Can you work these out from the model? Positions are in its coordinate system, mm. A direction names the side the tool comes from. Give positions to 0.01 mm unless a question says otherwise; leave off trailing zeros. Loops run counter-clockwise (first coordinate to the right, second up) from the corner with the lowest first, then second, coordinate; pieces in that order, holes last. Notation, with made-up numbers: (5.25, 29.5) - (13.25, 29.5) arc R25 cw to (13.25, 51.5) - close; hole circle Ø10 at (-22, -10). An arc over 180 degrees is marked (long way). Write item = value, one per line.
from build123d import *

# Parameters (mm, degrees)
SKETCH_31_W              = 56.5
SKETCH_31_H              = 38
EXTRUDE_11_DEPTH         = 4
SKETCH_32_W              = 4
SKETCH_32_H              = 38
EXTRUDE_12_DEPTH         = 29.5
SKETCH_33_W              = 16
SKETCH_33_H              = 38
EXTRUDE_13_DEPTH         = 4
SKETCH_34_W              = 15
SKETCH_34_H              = 4
EXTRUDE_14_DEPTH         = 29.5
HOLE_WIZARD_M2_5_1_D     = 2.9
HOLE_WIZARD_M2_5_1_DEPTH = 10
HOLE_WIZARD_M2_5_1_TIP   = 0.871247898
HOLE_WIZARD_M2_5_2_D     = 2.9
HOLE_WIZARD_M2_5_2_DEPTH = 10
HOLE_WIZARD_M2_5_2_TIP   = 0.871247898
HOLE_WIZARD_M2_5_3_D     = 2.9
HOLE_WIZARD_M2_5_3_DEPTH = 10
HOLE_WIZARD_M2_5_3_TIP   = 0.871247898
HOLE_WIZARD_M4_1_D       = 4.5
HOLE_WIZARD_M4_1_DEPTH   = 10
HOLE_WIZARD_M4_1_TIP     = 1.351936393
SKETCH_46_W              = 43
SKETCH_46_H              = 33.5
CUT_EXTRUDE_4_DEPTH      = 4


with BuildPart() as part:
    # 스케치31 → 보스-돌출11 (new body)
    with BuildSketch(Plane(origin=(0, 0, 0), x_dir=(1, 0, 0), z_dir=(0, 1, 0))):
        Rectangle(SKETCH_31_W, SKETCH_31_H)
    extrude(amount=EXTRUDE_11_DEPTH)

    # 스케치32 → 보스-돌출12 (add)
    with BuildSketch(Plane.XZ):
        with Locations((26.25, 0)):
            Rectangle(SKETCH_32_W, SKETCH_32_H)
        with Locations((-26.25, 0)):
            Rectangle(SKETCH_32_W, SKETCH_32_H)
    extrude(amount=EXTRUDE_12_DEPTH)

    # 스케치33 → 보스-돌출13 (add)
    with BuildSketch(Plane.XZ.offset(29.5)):
        with Locations((-36.25, 0)):
            Rectangle(SKETCH_33_W, SKETCH_33_H)
        with Locations((36.25, 0)):
            Rectangle(SKETCH_33_W, SKETCH_33_H)
    extrude(amount=-EXTRUDE_13_DEPTH)

    # 스케치34 → 보스-돌출14 (add)
    with BuildSketch(Plane.XZ):
        with Locations((-16.75, 17)):
            Rectangle(SKETCH_34_W, SKETCH_34_H)
    extrude(amount=EXTRUDE_14_DEPTH)

    # M2.5 여유 구멍1
    with Locations(Plane(origin=(0, 4, 0), x_dir=(1, 0, 0), z_dir=(0, 1, 0))):
        with Locations((8, 8), (8, -4), (-16, -4), (-16, 8)):
            Hole(HOLE_WIZARD_M2_5_1_D / 2, depth=HOLE_WIZARD_M2_5_1_DEPTH)
            with Locations((0, 0, -(HOLE_WIZARD_M2_5_1_DEPTH + HOLE_WIZARD_M2_5_1_TIP / 2))):  # 118° drill point
                Cone(0, HOLE_WIZARD_M2_5_1_D / 2, HOLE_WIZARD_M2_5_1_TIP, mode=Mode.SUBTRACT)

    # M2.5 여유 구멍2
    with Locations(Plane(origin=(28.25, 0, 0), x_dir=(0, 0, -1), z_dir=(1, 0, 0))):
        with Locations((-4, -7.25), (8, -7.25)):
            Hole(HOLE_WIZARD_M2_5_2_D / 2, depth=HOLE_WIZARD_M2_5_2_DEPTH)
            with Locations((0, 0, -(HOLE_WIZARD_M2_5_2_DEPTH + HOLE_WIZARD_M2_5_2_TIP / 2))):  # 118° drill point
                Cone(0, HOLE_WIZARD_M2_5_2_D / 2, HOLE_WIZARD_M2_5_2_TIP, mode=Mode.SUBTRACT)

    # M2.5 여유 구멍3
    with Locations(Plane.ZY.offset(28.25)):
        with Locations((4, -7.25), (-8, -7.25)):
            Hole(HOLE_WIZARD_M2_5_3_D / 2, depth=HOLE_WIZARD_M2_5_3_DEPTH)
            with Locations((0, 0, -(HOLE_WIZARD_M2_5_3_DEPTH + HOLE_WIZARD_M2_5_3_TIP / 2))):  # 118° drill point
                Cone(0, HOLE_WIZARD_M2_5_3_D / 2, HOLE_WIZARD_M2_5_3_TIP, mode=Mode.SUBTRACT)

    # M4 여유 구멍1
    with Locations(Plane(origin=(0, -25.5, 0), x_dir=(1, 0, 0), z_dir=(0, 1, 0))):
        with Locations((37.25, 10), (37.25, -10), (-37.25, -10), (-37.25, 10)):
            Hole(HOLE_WIZARD_M4_1_D / 2, depth=HOLE_WIZARD_M4_1_DEPTH)
            with Locations((0, 0, -(HOLE_WIZARD_M4_1_DEPTH + HOLE_WIZARD_M4_1_TIP / 2))):  # 118° drill point
                Cone(0, HOLE_WIZARD_M4_1_D / 2, HOLE_WIZARD_M4_1_TIP, mode=Mode.SUBTRACT)

    # 스케치46 → 컷-돌출4 (cut)
    with BuildSketch(Plane.XY.offset(19)):
        with Locations((22.75, -12.75)):
            Rectangle(SKETCH_46_W, SKETCH_46_H)
    extrude(amount=-CUT_EXTRUDE_4_DEPTH, mode=Mode.SUBTRACT)


solid = part.part
Q1. I need wall thicknesses on L1, parallel to Z at x = 8, y = 1; L2, parallel to Z at x = -37, y = -27; L3, parallel to X at y = 1.7, z = -8. Which ranges of each line are inside material? Lowest first, please.
Output:
L1 = -19 to -9.45, -6.55 to 2.55, 5.45 to 15
L2 = -19 to -12.24, -7.76 to 7.76, 12.24 to 19
L3 = -28.25 to -17.45, -14.55 to 6.55, 9.45 to 28.25
Q2. Imagine slicing it at B-B, the plane z = 4. Write out the boundary of the cut face in (x, y), then the cut area to 3 significant figures.
Output:
outline = (-44.25, -29.5) - (-24.25, -29.5) - (-24.25, -8.7) - (-28.25, -8.7) - (-28.25, -25.5) - (-44.25, -25.5) - close; (-28.25, -5.8) - (-24.25, -5.8) - (-24.25, 0) - (-17.45, 0) - (-17.45, 4) - (-28.25, 4) - close; (-14.55, 0) - (6.55, 0) - (6.55, 4) - (-14.55, 4) - close; (9.45, 0) - (24.25, 0) - (24.25, -5.8) - (28.25, -5.8) - (28.25, 4) - (9.45, 4) - close; (24.25, -29.5) - (44.25, -29.5) - (44.25, -25.5) - (28.25, -25.5) - (28.25, -8.7) - (24.25, -8.7) - close
area = 544 mm2
Q3. We'd pull the mould along X, two halves only. Please class faces 5 (the flat face through (0, 4, 0)), 6 (the flat face through (-44.25, -28, 0)), 7 (the cylindrical face through (36.04, -27.528, -11.897)): released by +X, released by -X, zero draft, split by the parting line, or undercut.
Output:
face_5 = zero draft
face_6 = released by -X
face_7 = undercut
Q4. Imagine slicing it at C-C, the plane y = -17.5. Write out the boundary of the cut face in (x, z).
Output:
outline = (-28.25, -19) - (-24.25, -19) - (-24.25, 15) - (-9.25, 15) - (-9.25, 19) - (-28.25, 19) - close; (24.25, -19) - (28.25, -19) - (28.25, 15) - (24.25, 15) - close
Q5. For pin 1 (1.7 mm diameter, centred on x = 8, z = 4, fed in from +Y); pin 2 (4.5 mm diameter, centred on y = -16.5, z = 18, fed in from +X); pin 3 (6 mm diameter, centred on x = -37.25, z = -10, fed in from +Y); pin 4 (9 mm diameter, centred on y = -11.5, z = -5.5, fed in from +X), each with a flat end and sliding along its axis, tell me the tip position at first contact or that it passes through.
Output:
pin_1 = through
pin_2 = -9.25
pin_3 = -25.5
pin_4 = 28.25
Q6. Which directions (+Z, -Z, +X, -X, +Y, -Y) give clear straight access to the entire face, cutting with the end or side of a thin tool? Please do faces 1 (the flat face through (-36, -25.5, 0)), 2 (the flat face through (-17, -15, 15)), 3 (the flat face through (24.25, -15, -2)), 4 (the flat face through (1.25, 2, 17)).
Output:
face_1 = +Z, -Z, -X, +Y
face_2 = -Z, -Y
face_3 = +Z, -Z, -Y
face_4 = +Z, +X, +Y, -Y
Q7. Imagine slicing it at D-D, the plane z = -4. Write out the boundary of the cut face in (x, y).
Output:
outline = (-44.25, -29.5) - (-24.25, -29.5) - (-24.25, 0) - (24.25, 0) - (24.25, -29.5) - (44.25, -29.5) - (44.25, -25.5) - (28.25, -25.5) - (28.25, 4) - (-28.25, 4) - (-28.25, -25.5) - (-44.25, -25.5) - close
Q8. Imagine slicing it at A-A, the plane x = 8. Write out the boundary of the cut face in (y, z), then the cut area to 3 significant figures.
Output:
outline = (0, -19) - (4, -19) - (4, -9.45) - (0, -9.45) - close; (0, -6.55) - (4, -6.55) - (4, 2.55) - (0, 2.55) - close; (0, 5.45) - (4, 5.45) - (4, 15) - (0, 15) - close
area = 113 mm2
